Verification items for the finished model (mm, model axes). Round coordinates to 2 decimals unless told otherwise and drop trailing zeros. Loops run counter-clockwise (first coordinate to the right, second up) from the corner with the lowest first, then second, coordinate; pieces in that order, holes last. Notation, with made-up numbers: M -1,4 L 45,4 A16 ccw 45,32 Z; hole C -4.75,50.25 d3. An arc over 180 degrees is marked long. Answer as CSV lines item,"result".
```python
from build123d import *

# Parameters (mm, degrees)
SKETCH1_W           = 609.6
SKETCH1_H           = 1219.2
BOSS_EXTRUDE1_DEPTH = 3.175
SKETCH2_R           = 29.21
CUT_EXTRUDE1_DEPTH  = 682.560914831
SKETCH3_R           = 1.5875
CUT_EXTRUDE2_DEPTH  = 682.560914831


with BuildPart() as part:
    # Sketch1 → Boss-Extrude1 (new body)
    with BuildSketch(Plane(origin=(0, 0, 0), x_dir=(0, 0, -1), z_dir=(1, 0, 0))):
        Rectangle(SKETCH1_W, SKETCH1_H)
    extrude(amount=BOSS_EXTRUDE1_DEPTH)

    # Sketch2 → Cut-Extrude1 (cut, through all)
    with BuildSketch(Plane(origin=(3.175, 0, 0), x_dir=(0, 0, -1), z_dir=(1, 0, 0))):
        with Locations((-50.8, -431.8)):
            Circle(SKETCH2_R)
        with Locations((50.8, -431.8)):
            Circle(SKETCH2_R)
    cut_extrude1 = extrude(amount=-CUT_EXTRUDE1_DEPTH, mode=Mode.SUBTRACT)

    # Sketch3 → Cut-Extrude2 (cut, through all)
    with BuildSketch(Plane(origin=(3.175, 0, 0), x_dir=(0, 0, -1), z_dir=(1, 0, 0))):
        with Locations((-88.9, -368.3)):
            Circle(SKETCH3_R)
        with Locations((88.9, -368.3)):
            Circle(SKETCH3_R)
        with Locations((-88.9, -495.3)):
            Circle(SKETCH3_R)
        with Locations((88.9, -495.3)):
            Circle(SKETCH3_R)
    cut_extrude2 = extrude(amount=-CUT_EXTRUDE2_DEPTH, mode=Mode.SUBTRACT)

    # Mirror1: Cut-Extrude1, Cut-Extrude2 across plane
    add(cut_extrude1.mirror(Plane.ZX), mode=Mode.SUBTRACT)
    add(cut_extrude2.mirror(Plane.ZX), mode=Mode.SUBTRACT)


solid = part.part
```
1) Draft check along Z on faces 1 (the flat face through (3.175, 9, 4)), 2 (the cylindrical face through (1.61, -412.06, -29.27)). Enter one of: +Z half, -Z half, draft (parallel to the pull), parting line (faces both ways), or undercut.
Here are the results:
face 1,"draft"
face 2,"undercut"
2) Material ranges on probe 1 along Z at (x, y) = (2.2, -368.3); probe 2 along Y at (x, z) = (1.15, 50.8); probe 3 along Y at (x, z) = (1.65, -88.9), recorded low to high.
Here are the results:
probe 1,"z = -304.8 to -90.49, -87.31 to 87.31, 90.49 to 304.8"
probe 2,"y = -609.6 to -461.01, -402.59 to 402.59, 461.01 to 609.6"
probe 3,"y = -609.6 to -496.89, -493.71 to -369.89, -366.71 to 366.71, 369.89 to 493.71, 496.89 to 609.6"
3) Section check A-A (z = 50.8). Record the cut outline in (x, y) (3 decimals).
Here are the results:
outline,"M 0,-609.6 L 3.175,-609.6 L 3.175,-461.01 L 0,-461.01 Z; M 0,-402.59 L 3.175,-402.59 L 3.175,402.59 L 0,402.59 Z; M 0,461.01 L 3.175,461.01 L 3.175,609.6 L 0,609.6 Z"
